from build123d import *

# Parameters (mm, degrees)
CROQUIS1_R                 = 12.7
SALIENTE_EXTRUIR1_DEPTH    = 12.5
CROQUIS2_R                 = 4.5
SALIENTE_EXTRUIR2_DEPTH    = 24.5
CORTAR_EXTRUIR1_DEPTH      = 31.378117124
CORTAR_EXTRUIR1_DEPTH_BACK = 31.378117124
CROQUIS3_R                 = 2.460715963


with BuildPart() as part:
    # Croquis1 → Saliente-Extruir1 (new, symmetric)
    with BuildSketch(Plane(origin=(0, 0, 0), x_dir=(1, 0, 0), z_dir=(0, 1, 0))):
        with Locations(Location((0, 0, 0), (0, 0, 270))):
            Circle(CROQUIS1_R)
    extrude(amount=SALIENTE_EXTRUIR1_DEPTH, both=True)

    # Croquis2 → Saliente-Extruir2 (add, symmetric)
    with BuildSketch(Plane(origin=(0, 0, 0), x_dir=(1, 0, 0), z_dir=(0, 1, 0))):
        with Locations(Location((0, 0, 0), (0, 0, 270))):
            Circle(CROQUIS2_R)
    extrude(amount=SALIENTE_EXTRUIR2_DEPTH, both=True)

    # Croquis3 → Cortar-Extruir1 (cut, two sides: drawn at the far end of the back side and taken through both)
    with BuildSketch(Plane(origin=(0, 0, 0), x_dir=(1, 0, 0), z_dir=(0, 1, 0)).offset(-CORTAR_EXTRUIR1_DEPTH_BACK)):
        with Locations(Location((0, 0, 0), (0, 0, 270))):
            Circle(CROQUIS3_R)
    extrude(amount=CORTAR_EXTRUIR1_DEPTH + CORTAR_EXTRUIR1_DEPTH_BACK, mode=Mode.SUBTRACT)


solid = part.part
Can you work these out from the model? Positions are in its coordinate system, mm. A direction names the side the tool comes from. Give positions to 0.01 mm unless a question says otherwise; leave off trailing zeros. Write each loop counter-clockwise with the first axis right and the second up, starting at its lowest first coordinate (ties: lowest second). Pieces come first, ordered by that corner, then holes. Notation, with made-up numbers: (82, 80) -> (140, 80) arc R7 cw to (140, 90) -> close; hole circle Ø9 at (28.5, 61.25). An arc over 180 degrees is marked (long way). Answer as a JSON object with one key per item and string values. Group by question number.
Item 1: Suppose I cut it at A-A (z = 0). Please give me the cut outline in (x, y).
Item 2: Suppose I cut it at C-C (y = 4). Please give me the cut outline in (x, z), plus the area to 3 significant figures.
Item 3: We'd pull the mould along X, two halves only. Please class faces 4 (the face through (1.352, 18.584, 4.292)), 5 (the face through (0, -12.5, 5)), 6 (the face through (-2.2, -0.3, 1.1)): +X half, -X half, draft (parallel to the pull), parting line (faces both ways), or undercut.
Item 4: Suppose I cut it at D-D (x = -3). Please give me the cut outline in (y, z), plus the area to 3 significant figures.
Item 5: Suppose I cut it at B-B (x = 0). Please give me the cut outline in (y, z).
Item 6: For faces 1 (the face through (1.352, -18.416, 4.292)), 2 (the face through (-2, 24.5, 2)), 3 (the face through (0, 12.5, 5)), which set-ups out of +Z, -Z, +X, -X, +Y, -Y let a thin tool reach every point of the face, with its end or its side?
Item 7: Please list where these lines run through material, in increasing order: line 1 (X direction, y = -11, z = 0); line 2 (Y direction, x = 1.5, z = -9.75); line 3 (X direction, y = 8.5, z = 1.25). Write a range as [from, to].
Item 8: I'm going to push flat-ended pins straight in: P1, Ø1, axis at x = -4, y = 6, coming from the -Z side; P2, Ø4, axis at y = -5.5, z = 4, coming from the +X side; P3, Ø6, axis at x = -4.5, y = 5.5, coming from the +Z side. Where does each tip first touch, or does it pass through?
Findings:
{
 "1": {"outline": "(-12.7, -12.5) -> (-4.5, -12.5) -> (-4.5, -24.5) -> (-2.46, -24.5) -> (-2.46, 24.5) -> (-4.5, 24.5) -> (-4.5, 12.5) -> (-12.7, 12.5) -> close; (2.46, -24.5) -> (4.5, -24.5) -> (4.5, -12.5) -> (12.7, -12.5) -> (12.7, 12.5) -> (4.5, 12.5) -> (4.5, 24.5) -> (2.46, 24.5) -> close"},
 "2": {"outline": "circle Ø25.4 at (0, 0); hole circle Ø4.92 at (0, 0)", "area": "488 mm²"},
 "3": {"face 4": "parting line", "face 5": "draft", "face 6": "undercut"},
 "4": {"outline": "(-24.5, -3.35) -> (-12.5, -3.35) -> (-12.5, -12.34) -> (12.5, -12.34) -> (12.5, -3.35) -> (24.5, -3.35) -> (24.5, 3.35) -> (12.5, 3.35) -> (12.5, 12.34) -> (-12.5, 12.34) -> (-12.5, 3.35) -> (-24.5, 3.35) -> close", "area": "778 mm²"},
 "5": {"outline": "(-24.5, -4.5) -> (-12.5, -4.5) -> (-12.5, -12.7) -> (12.5, -12.7) -> (12.5, -4.5) -> (24.5, -4.5) -> (24.5, -2.46) -> (-24.5, -2.46) -> close; (-24.5, 2.46) -> (24.5, 2.46) -> (24.5, 4.5) -> (12.5, 4.5) -> (12.5, 12.7) -> (-12.5, 12.7) -> (-12.5, 4.5) -> (-24.5, 4.5) -> close"},
 "6": {"face 1": "-Y", "face 2": "+Z, -Z, +X, -X, +Y", "face 3": "+Y"},
 "7": {"line 1": "x = [-12.7, -2.46], [2.46, 12.7]", "line 2": "y = [-12.5, 12.5]", "line 3": "x = [-12.64, -2.12], [2.12, 12.64]"},
 "8": {"P1": "stops at z = -12.21", "P2": "stops at x = 12.54", "P3": "stops at z = 12.61"}
}
